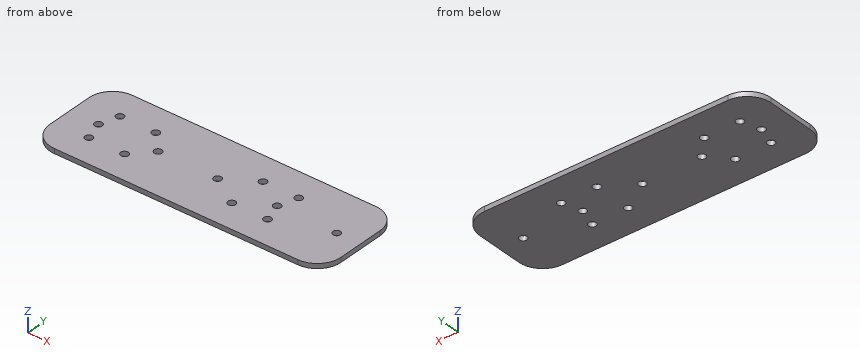
```python
from build123d import *

# Parameters (mm, degrees)
SKETCH_1_W          = 140
SKETCH_1_H          = 40
SKETCH_1_R          = 1.6
EXTRUDE_1_DEPTH     = 2
FILLET_1_R          = 10
SKETCH_2_W          = 24.439336454
SKETCH_2_H          = 40
CUT_EXTRUDE_1_DEPTH = 10
FILLET_2_R          = 10


with BuildPart() as part:
    # 草图1 → 凸台-拉伸1 (new body)
    with BuildSketch(Plane.XY):
        Rectangle(SKETCH_1_W, SKETCH_1_H)
        with Locations((37.5, 8)):
            Circle(SKETCH_1_R, mode=Mode.SUBTRACT)
        with Locations((37.5, -8)):
            Circle(SKETCH_1_R, mode=Mode.SUBTRACT)
        with Locations((22.5, -8)):
            Circle(SKETCH_1_R, mode=Mode.SUBTRACT)
        with Locations((22.5, 8)):
            Circle(SKETCH_1_R, mode=Mode.SUBTRACT)
        with Locations((-22.5, -8)):
            Circle(SKETCH_1_R, mode=Mode.SUBTRACT)
        with Locations((-37.5, -8)):
            Circle(SKETCH_1_R, mode=Mode.SUBTRACT)
        with Locations((-22.5, 8)):
            Circle(SKETCH_1_R, mode=Mode.SUBTRACT)
        with Locations((-37.5, 8)):
            Circle(SKETCH_1_R, mode=Mode.SUBTRACT)
        with Locations((60, 0)):
            Circle(SKETCH_1_R, mode=Mode.SUBTRACT)
        with Locations((35, 0)):
            Circle(SKETCH_1_R, mode=Mode.SUBTRACT)
        with Locations((10, 0)):
            Circle(SKETCH_1_R, mode=Mode.SUBTRACT)
        with Locations((-15, 0)):
            Circle(SKETCH_1_R, mode=Mode.SUBTRACT)
        with Locations((-40, 0)):
            Circle(SKETCH_1_R, mode=Mode.SUBTRACT)
    extrude(amount=EXTRUDE_1_DEPTH)

    # 圆角1
    fillet_1_edges = [part.edges().sort_by_distance(p)[0] for p in [
        (70, -20, 1),
        (-70, -20, 1),
        (-70, 20, 1),
        (70, 20, 1),
    ]]
    fillet(fillet_1_edges, radius=FILLET_1_R)

    # 草图2 → 切除-拉伸1 (cut)
    with BuildSketch(Plane.XY.offset(2)):
        with Locations((-64.426426614, 0)):
            Rectangle(SKETCH_2_W, SKETCH_2_H)
    extrude(amount=-CUT_EXTRUDE_1_DEPTH, mode=Mode.SUBTRACT)

    # 圆角2
    fillet_2_edges = [part.edges().sort_by_distance(p)[0] for p in [
        (-52.206758387, 20, 1),
        (-52.206758387, -20, 1),
    ]]
    fillet(fillet_2_edges, radius=FILLET_2_R)


solid = part.part
```
Input: part model. Units: mm. Frame: model coordinates. Round coordinates to 2 decimals unless told otherwise and drop trailing zeros. Order: outer loops, then holes, each group sorted by start corner. A loop starts at its lowest first (then second) coordinate and runs counter-clockwise, first axis right, second up. Notation, with made-up numbers: (-28, 50) - (15, 50) arc R27 cw to (15, 78) - close; hole circle Ø4 at (-18, -25.5). An arc over 180 degrees is marked (long way). Answer in a Markdown table with one row per item.
Item 1: Section query D-D (x = -15). Return the cut outline in (y, z).
Model answer:
| item | result |
|---|---|
| outline | (-20, 0) - (-1.6, 0) - (-1.6, 2) - (-20, 2) - close; (1.6, 0) - (20, 0) - (20, 2) - (1.6, 2) - close |
Item 2: Line query: line 1 (Y direction, x = -37.5, z = 0.6); line 2 (Y direction, x = -15, z = 0.55); line 3 (X direction, y = -7, z = 0.2). Output: solid intervals per line, ascending.
Model answer:
| item | result |
|---|---|
| line 1 | y = -20 to -9.6, -6.4 to 6.4, 9.6 to 20 |
| line 2 | y = -20 to -1.6, 1.6 to 20 |
| line 3 | x = -52.21 to -38.75, -36.25 to -23.75, -21.25 to 21.25, 23.75 to 36.25, 38.75 to 70 |
Item 3: Section query B-B (x = 22.5). Return the cut outline in (y, z), then the cut area to 3 significant figures.
Model answer:
| item | result |
|---|---|
| outline | (-20, 0) - (-9.6, 0) - (-9.6, 2) - (-20, 2) - close; (-6.4, 0) - (6.4, 0) - (6.4, 2) - (-6.4, 2) - close; (9.6, 0) - (20, 0) - (20, 2) - (9.6, 2) - close |
| area | 67.2 mm² |
Item 4: Section query C-C (y = -8). Return the cut outline in (x, z), then the cut area to 3 significant figures.
Model answer:
| item | result |
|---|---|
| outline | (-52.21, 0) - (-39.1, 0) - (-39.1, 2) - (-52.21, 2) - close; (-35.9, 0) - (-24.1, 0) - (-24.1, 2) - (-35.9, 2) - close; (-20.9, 0) - (20.9, 0) - (20.9, 2) - (-20.9, 2) - close; (24.1, 0) - (35.9, 0) - (35.9, 2) - (24.1, 2) - close; (39.1, 0) - (70, 0) - (70, 2) - (39.1, 2) - close |
| area | 219 mm² |
Item 5: Section query A-A (y = 0). Return the cut outline in (x, z), then the cut area to 3 significant figures.
Model answer:
| item | result |
|---|---|
| outline | (-52.21, 0) - (-41.6, 0) - (-41.6, 2) - (-52.21, 2) - close; (-38.4, 0) - (-16.6, 0) - (-16.6, 2) - (-38.4, 2) - close; (-13.4, 0) - (8.4, 0) - (8.4, 2) - (-13.4, 2) - close; (11.6, 0) - (33.4, 0) - (33.4, 2) - (11.6, 2) - close; (36.6, 0) - (58.4, 0) - (58.4, 2) - (36.6, 2) - close; (61.6, 0) - (70, 0) - (70, 2) - (61.6, 2) - close |
| area | 212 mm² |
